Build history of the part. All positions in model axes, mm. A direction names the side the tool comes from. Coordinates: 2 decimals unless noted, no trailing zeros. Loops run counter-clockwise (first coordinate to the right, second up) from the corner with the lowest first, then second, coordinate; pieces in that order, holes last.
Item 1: Cut at A-A (z = -10). List the corners of the cut face in (x, y).
Item 2: Cut at B-B (x = -6). List the corners of the cut face in (y, z).
Item 3: Mould opens along Z. For faces 3 (the face through (-4, 1, -12.395)), 4 (the face through (-4, 1, 12.605)), 5 (the face through (-4, 0, 0)), 6 (the face through (-15.272, 1, -10)) say: released by +Z, released by -Z, zero draft, split by the parting line, or undercut.
Item 4: 3-axis set-ups, long thin cutter, end or side, ignore diameter. For faces 1 (the face through (-4, 1, -8.895)), 2 (the face through (21.778, 1, 0)): which of +Z, -Z, +X, -X, +Y, -Y reach the whole face in a straight line?
Item 5: Drill centre lines: line 1 along Z through (x, y) = (-2, 0.4); line 2 along X through (y, z) = (0.15, -10.25). Where is each one in solid material? Low to high.
Item 6: Cut at C-C (y = 1.25). List the corners of the cut face in (x, z), and give its area (3 significant figures).
from build123d import *

# Parameters (mm, degrees)
SKETCH1_W               = 51
SKETCH1_H               = 25
BOSS_EXTRUDE1_DEPTH     = 2
CUT_EXTRUDE1_DEPTH      = 32.886989955
CUT_EXTRUDE1_DEPTH_BACK = 32.886989955
SKETCH3_W               = 13.1
SKETCH3_H               = 2.1
SKETCH4_W               = 23.1
SKETCH4_H               = 2.1
CUT_EXTRUDE2_DEPTH      = 10


with BuildPart() as part:
    # Sketch1 → Boss-Extrude1 (new body)
    with BuildSketch(Plane(origin=(0, 0, 0), x_dir=(1, 0, 0), z_dir=(0, 1, 0))):
        with Locations((-3.721556886, -0.104790419)):
            Rectangle(SKETCH1_W, SKETCH1_H)
    extrude(amount=BOSS_EXTRUDE1_DEPTH)

    # Sketch3 → Cut-Extrude1 (cut, two sides: drawn at the far end of the back side and taken through both)
    with BuildSketch(Plane(origin=(0, 2, 0), x_dir=(1, 0, 0), z_dir=(0, 1, 0)).offset(-CUT_EXTRUDE1_DEPTH_BACK)):
        with Locations((-3.721556886, 9.945209581)):
            Rectangle(SKETCH3_W, SKETCH3_H)
    extrude(amount=CUT_EXTRUDE1_DEPTH + CUT_EXTRUDE1_DEPTH_BACK, mode=Mode.SUBTRACT)

    # Sketch4 → Cut-Extrude2 (cut)
    with BuildSketch(Plane(origin=(0, 2, 0), x_dir=(1, 0, 0), z_dir=(0, 1, 0))):
        with Locations((-3.721556886, 9.945209581)):
            Rectangle(SKETCH4_W, SKETCH4_H)
    extrude(amount=-CUT_EXTRUDE2_DEPTH, mode=Mode.SUBTRACT)


solid = part.part
Filled sheet:
1. outline: (-29.22, 0) - (-15.27, 0) - (-15.27, 2) - (-29.22, 2) - close; (7.83, 0) - (21.78, 0) - (21.78, 2) - (7.83, 2) - close
2. outline: (0, -12.4) - (2, -12.4) - (2, -11) - (0, -11) - close; (0, -8.9) - (2, -8.9) - (2, 12.6) - (0, 12.6) - close
3. face 3: released by -Z
3. face 4: released by +Z
3. face 5: zero draft
3. face 6: undercut
4. face 1: +Y, -Y
4. face 2: +Z, -Z, +X, +Y, -Y
5. line 1: z = -12.4 to -11, -8.9 to 12.6
5. line 2: x = -29.22 to -15.27, 7.83 to 21.78
6. outline: (-29.22, -12.4) - (21.78, -12.4) - (21.78, 12.6) - (-29.22, 12.6) - close; hole (-15.27, -11) - (7.83, -11) - (7.83, -8.9) - (-15.27, -8.9) - close
6. area: 1,230 mm2
